Input: part model. Units: mm. Frame: model coordinates. Give positions to 0.01 mm unless a question says otherwise; leave off trailing zeros. Write each loop counter-clockwise with the first axis right and the second up, starting at its lowest first coordinate (ties: lowest second). Pieces come first, ordered by that corner, then holes. Notation, with made-up numbers: (31.25, 71.25) -> (43.25, 71.25) arc R24 cw to (43.25, 103.25) -> close; hole circle Ø6 at (19.25, -14). An arc over 180 degrees is marked (long way). Return JSON: item names as keys, results as strings. Group by question number.
Item 1: Line query: line 1 (Z direction, x = -85.5, y = 1); line 2 (X direction, y = 2.5, z = -23); line 3 (X direction, y = 2.5, z = -78.5). Output: solid intervals per line, ascending. Write a range as [from, to].
Item 2: Pin query (flat end, axial travel): P1, Ø3, axis at y = 1, z = -15, coming from the -X side; P2, Ø1, axis at y = 2, z = -96, coming from the -X side. Return the tip coordinate at first contact, or that it passes through.
Item 3: Section A-A, the plane y = 5. Return loops of the section in (x, z), then the cut area to 3 significant figures.
Item 4: Section C-C, the plane x = -63. Return loops of the section in (y, z).
Item 5: Section B-B, the plane z = -25.5. Return loops of the section in (x, y).
from build123d import *

# Parameters (mm, degrees)
BOSS_EXTRU_1_DEPTH = 6.35


with BuildPart() as part:
    # Esquisse1 → Boss.-Extru.1 (new body)
    with BuildSketch(Plane(origin=(0, 0, 0), x_dir=(1, 0, 0), z_dir=(0, 1, 0))):
        Polygon((-101.6, 139.7), (-101.6, 127), (-74.6125, 127), (-31.75, 0), (31.75, 0), (74.6125, 127), (101.6, 127), (101.6, 139.7), align=None)
    extrude(amount=BOSS_EXTRU_1_DEPTH)


solid = part.part
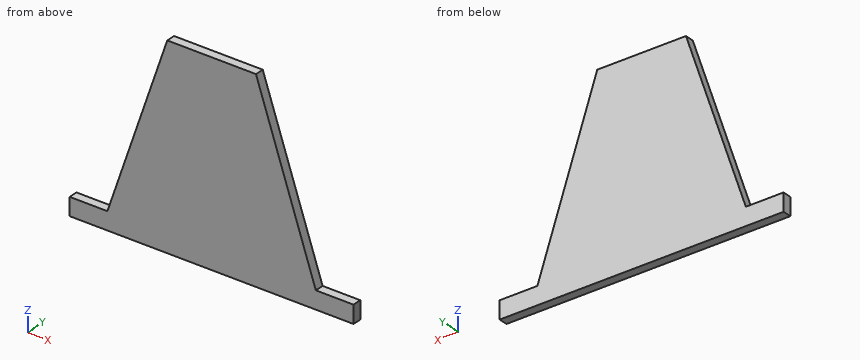
Answer below:
{
 "1": {"line 1": "z = [-139.7, -127]", "line 2": "x = [-39.51, 39.51]", "line 3": "x = [-58.24, 58.24]"},
 "2": {"P1": "stops at x = -37.32", "P2": "stops at x = -64.32"},
 "3": {"outline": "(-101.6, -139.7) -> (101.6, -139.7) -> (101.6, -127) -> (74.61, -127) -> (31.75, 0) -> (-31.75, 0) -> (-74.61, -127) -> (-101.6, -127) -> close", "area": "16,100 mm2"},
 "4": {"outline": "(0, -139.7) -> (6.35, -139.7) -> (6.35, -92.59) -> (0, -92.59) -> close"},
 "5": {"outline": "(-40.36, 0) -> (40.36, 0) -> (40.36, 6.35) -> (-40.36, 6.35) -> close"}
}
